from build123d import *
from OCP.BRepFilletAPI import BRepFilletAPI_MakeChamfer

# Parameters (mm, degrees)
SKETCH2_W           = 51.63
SKETCH2_H           = 51.63
SKETCH2_W_2         = 610
SKETCH2_H_2         = 6.35
BOSS_EXTRUDE1_DEPTH = 30
SKETCH2_4_W         = 630
SKETCH2_4_H         = 6.2
BOSS_EXTRUDE3_DEPTH = 3
FILLET2_R           = 3
CHAMFER1_SIZE       = 30
CHAMFER1_SIZE_2     = 5.289809421
CHAMFER2_SIZE       = 30
CHAMFER2_SIZE_2     = 5.289809421
SKETCH2_7_W         = 638
SKETCH2_7_H         = 26.35
SKETCH2_7_W_2       = 610
SKETCH2_7_H_2       = 6.35
BOSS_EXTRUDE5_DEPTH = 30


with BuildPart() as part:
    # Sketch2 → Boss-Extrude1 (new body)
    with BuildSketch(Plane(origin=(0, 0, 0), x_dir=(1, 0, 0), z_dir=(0, 1, 0))):
        Polygon((-350, -38.442), (-350, -65), (350, -65), (350, -38.442), (320, -38.442), (320, -15.674), (350, -15.674), (350, 15.674), (320, 15.674), (320, 38.442), (350, 38.442), (350, 65), (-350, 65), (-350, 38.442), (-320, 38.442), (-320, 15.674), (-350, 15.674), (-350, -15.674), (-320, -15.674), (-320, -38.442), align=None)
        with Locations((0, 4.815)):
            Rectangle(SKETCH2_W, SKETCH2_H, mode=Mode.SUBTRACT)
        with Locations((0, 51.825)):
            Rectangle(SKETCH2_W_2, SKETCH2_H_2, mode=Mode.SUBTRACT)
    extrude(amount=-BOSS_EXTRUDE1_DEPTH)

    # Sketch2<4> → Boss-Extrude3 (add)
    with BuildSketch(Plane(origin=(0, 0, 0), x_dir=(1, 0, 0), z_dir=(0, 1, 0))):
        with Locations((0, -51.56)):
            Rectangle(SKETCH2_4_W, SKETCH2_4_H)
    extrude(amount=BOSS_EXTRUDE3_DEPTH)

    # Fillet2
    fillet2_edges = [part.edges().sort_by_distance(p)[0] for p in [
        (0, 3, 48.46),
        (0, 3, 54.66),
    ]]
    fillet(fillet2_edges, radius=FILLET2_R - 0.0001)  # a hair under: the kernel refuses the full size

    # Chamfer1
    chamfer1_edges_1 = [part.edges().sort_by_distance(p)[0] for p in [
        (-335, -30, 15.674),
    ]]
    chamfer1_side_1 = [part.faces().sort_by_distance(p)[0] for p in [
        (-335, -29.894203812, 15.674),
    ]]
    chamfer1_edges_2 = [part.edges().sort_by_distance(p)[0] for p in [
        (-335, -30, -38.442),
    ]]
    chamfer1_side_2 = [part.faces().sort_by_distance(p)[0] for p in [
        (-335, -29.894203812, -38.442),
    ]]
    chamfer1_edges_3 = [part.edges().sort_by_distance(p)[0] for p in [
        (335, -30, -15.674),
    ]]
    chamfer1_side_3 = [part.faces().sort_by_distance(p)[0] for p in [
        (335, -29.894203812, -15.674),
    ]]
    chamfer1_edges_4 = [part.edges().sort_by_distance(p)[0] for p in [
        (335, -30, 38.442),
    ]]
    chamfer1_side_4 = [part.faces().sort_by_distance(p)[0] for p in [
        (335, -29.894203812, 38.442),
    ]]
    chamfer1 = BRepFilletAPI_MakeChamfer(part.part.solid().wrapped)
    for e in chamfer1_edges_1:
        chamfer1.Add(CHAMFER1_SIZE - 0.0001, CHAMFER1_SIZE_2 - 0.0001, e.wrapped, chamfer1_side_1[0].wrapped)
    for e in chamfer1_edges_2:
        chamfer1.Add(CHAMFER1_SIZE - 0.0001, CHAMFER1_SIZE_2 - 0.0001, e.wrapped, chamfer1_side_2[0].wrapped)
    for e in chamfer1_edges_3:
        chamfer1.Add(CHAMFER1_SIZE - 0.0001, CHAMFER1_SIZE_2 - 0.0001, e.wrapped, chamfer1_side_3[0].wrapped)
    for e in chamfer1_edges_4:
        chamfer1.Add(CHAMFER1_SIZE - 0.0001, CHAMFER1_SIZE_2 - 0.0001, e.wrapped, chamfer1_side_4[0].wrapped)
    add(Compound.cast(chamfer1.Shape()), mode=Mode.REPLACE)  # a hair under: the kernel refuses the full size

    # Chamfer2
    chamfer2_edges_1 = [part.edges().sort_by_distance(p)[0] for p in [
        (-335, -30, 38.442),
    ]]
    chamfer2_side_1 = [part.faces().sort_by_distance(p)[0] for p in [
        (-335, -29.894203812, 38.442),
    ]]
    chamfer2_edges_2 = [part.edges().sort_by_distance(p)[0] for p in [
        (-335, -30, -15.674),
    ]]
    chamfer2_side_2 = [part.faces().sort_by_distance(p)[0] for p in [
        (-335, -29.894203812, -15.674),
    ]]
    chamfer2_edges_3 = [part.edges().sort_by_distance(p)[0] for p in [
        (335, -30, -38.442),
    ]]
    chamfer2_side_3 = [part.faces().sort_by_distance(p)[0] for p in [
        (335, -29.894203812, -38.442),
    ]]
    chamfer2_edges_4 = [part.edges().sort_by_distance(p)[0] for p in [
        (335, -30, 15.674),
    ]]
    chamfer2_side_4 = [part.faces().sort_by_distance(p)[0] for p in [
        (335, -29.894203812, 15.674),
    ]]
    chamfer2 = BRepFilletAPI_MakeChamfer(part.part.solid().wrapped)
    for e in chamfer2_edges_1:
        chamfer2.Add(CHAMFER2_SIZE - 0.0001, CHAMFER2_SIZE_2 - 0.0001, e.wrapped, chamfer2_side_1[0].wrapped)
    for e in chamfer2_edges_2:
        chamfer2.Add(CHAMFER2_SIZE - 0.0001, CHAMFER2_SIZE_2 - 0.0001, e.wrapped, chamfer2_side_2[0].wrapped)
    for e in chamfer2_edges_3:
        chamfer2.Add(CHAMFER2_SIZE - 0.0001, CHAMFER2_SIZE_2 - 0.0001, e.wrapped, chamfer2_side_3[0].wrapped)
    for e in chamfer2_edges_4:
        chamfer2.Add(CHAMFER2_SIZE - 0.0001, CHAMFER2_SIZE_2 - 0.0001, e.wrapped, chamfer2_side_4[0].wrapped)
    add(Compound.cast(chamfer2.Shape()), mode=Mode.REPLACE)  # a hair under: the kernel refuses the full size

    # Sketch2<7> → Boss-Extrude5 (add)
    with BuildSketch(Plane(origin=(0, 0, 0), x_dir=(1, 0, 0), z_dir=(0, 1, 0))):
        with Locations((0, 51.825)):
            Rectangle(SKETCH2_7_W, SKETCH2_7_H)
        with Locations((0, 51.825)):
            Rectangle(SKETCH2_7_W_2, SKETCH2_7_H_2, mode=Mode.SUBTRACT)
    extrude(amount=BOSS_EXTRUDE5_DEPTH)


solid = part.part
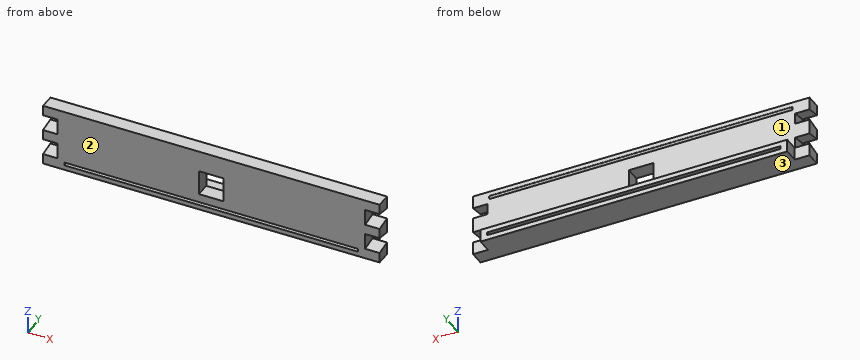
The model under review builds one solid part; all positions refer to its coordinate system, in mm. Face numbers are marked on the shaded views. Round coordinates to 2 decimals unless told otherwise and drop trailing zeros. Order: outer loops, then holes, each group sorted by start corner. A loop starts at its lowest first (then second) coordinate and runs counter-clockwise, first axis right, second up. Notation, with made-up numbers: (-40, -19.5) -> (16, -19.5) arc R37 cw to (16, 16.5) -> close; hole circle Ø7 at (-39.5, 46). An arc over 180 degrees is marked (long way). Use CSV: the item, a comma, the result in double quotes. Start each with the question number.
(1) Consider section D-D on y = -8. Write out the cut boundary in (x, z) (3 decimals), and give its area (3 significant figures).
(2) Mouldability with a two-part tool opening along Z and no side actions: class the marked faces 1, 2 and 3 as pulls with the +Z half, pulls with the -Z half, needs draft (parallel to the pull), parting line crosses it, or undercut.
(3) Wall thickness on probe 1 along X at (y, z) = (-2, -52); probe 2 along X at (y, z) = (-20.5, -22) (3 decimals); probe 3 along Z at (x, y) = (-222, -18.5): over which ranges is each line inside the solid? List them lowest first. Write a range as from..to.
(4) Consider section C-C on z = 27. Write out the cut boundary in (x, y).
(5) Insertion check: pin 1 (9 mm diameter, centred on y = -10, z = -34.5, fed in from +X); pin 2 (1 mm diameter, centred on y = -1, z = 20, fed in from -X); pin 3 (2.5 mm diameter, centred on y = 2, z = 51.5, fed in from -X); pin 4 (10 mm diameter, centred on y = 6, z = 11.5, fed in from -X). Each pin has a flat end and moves straight along its axis. Give the tip position at first contact, or say it passes through.
(6) Consider section B-B on y = 24. Write out the cut boundary in (x, z).
Responses:
1,outline,"(-350, -65) -> (350, -65) -> (350, -39.853) -> (320, -39.853) -> (320, -14.263) -> (350, -14.263) -> (350, 14.263) -> (320, 14.263) -> (320, 39.853) -> (350, 39.853) -> (350, 65) -> (-350, 65) -> (-350, 39.853) -> (-320, 39.853) -> (-320, 14.263) -> (-350, 14.263) -> (-350, -14.263) -> (-320, -14.263) -> (-320, -39.853) -> (-350, -39.853) -> close; hole (-305, -55) -> (305, -55) -> (305, -48.65) -> (-305, -48.65) -> close; hole (-25.815, -30.63) -> (25.815, -30.63) -> (25.815, 21) -> (-25.815, 21) -> close"
1,area,"81,400 mm²"
2,face 1,"undercut"
2,face 2,"needs draft"
2,face 3,"pulls with the -Z half"
3,probe 1,"-350..-305, 305..350"
3,probe 2,"-320..-25.815, 25.815..320"
3,probe 3,"-65..-55, -48.65..65"
4,outline,"(-320, -30) -> (320, -30) -> (320, 0) -> (-320, 0) -> close"
5,pin 1,"x = 320"
5,pin 2,"x = -320"
5,pin 3,"x = -315"
5,pin 4,"through"
6,outline,"(-319, -65) -> (319, -65) -> (319, -38.65) -> (-319, -38.65) -> close; hole (-305, -55) -> (305, -55) -> (305, -48.65) -> (-305, -48.65) -> close"
